The listing builds one solid part. Answer for the finished solid, in the listing's coordinates (mm). A direction names the side the tool comes from. Round coordinates to 2 decimals unless told otherwise and drop trailing zeros. Write each loop counter-clockwise with the first axis right and the second up, starting at its lowest first coordinate (ties: lowest second). Pieces come first, ordered by that corner, then holes. Notation, with made-up numbers: (89.5, -15) - (116.5, -15) arc R17 cw to (116.5, -3) - close; hole circle Ø10 at (24.25, -30). An arc over 180 degrees is marked (long way). Return JSON: item names as keys, results as strings. Group by question number.
(1) Which of the six approach directions +Z, -Z, +X, -X, +Y, -Y give full straight-line access (tool end or side, diameter ignored) to faces 1 (the cylindrical face through (17.161, 2.718, 4.213)), 2 (the cylindrical face through (-8.76, 1.535, -17.483)), 3 (the flat face through (-6, -1, 15))?
(2) Section A-A, the plane z = -22.5 is taken. Write down the section's boundary in (x, y).
(3) Determine the mould class of faces 4 (the flat face through (36, 0, 0)), 5 (the flat face through (-28, 0, 22)), 6 (the flat face through (-36, 0, 0)) for opening direction X: +X half, -X half, draft (parallel to the pull), parting line (faces both ways), or undercut.
(4) Section D-D, the plane z = 0 is taken. Write down the section's boundary in (x, y).
(5) Each of these flat-tipped pins is pushed along its axis until it touches: pin 1 (5.5 mm diameter, centred on x = 22.5, z = 15.5, fed in from -Y); pin 2 (2.5 mm diameter, centred on x = -32, z = -1, fed in from +Y); pin 3 (13 mm diameter, centred on x = -31, z = 22.5, fed in from +Y); pin 4 (6.5 mm diameter, centred on x = 3, z = -1.5, fed in from +Y). Where does it stop, or does it pass through?
(6) Find the intervals of material crossed by line 1 along Z through (x, y) = (-31, 2.85); line 2 along X through (y, z) = (2.1, -15.5); line 3 along Z through (x, y) = (-31, -1.3), in increasing order. Write a range as [from, to].
(7) Section C-C, the plane x = 7 is taken. Write down the section's boundary in (y, z), then the cut area to 3 significant figures.
(8) Section B-B, the plane y = -2 is taken. Give the number of separate pieces and of enclosed holes in the cut face, then the cut area to 3 significant figures.
```python
from build123d import *

# Parameters (mm, degrees)
SKETCH_1_W                = 72
SKETCH_1_H                = 65
EXTRUDE_1_DEPTH           = 4
HOLE_WIZARD_1_D           = 5.5
HOLE_WIZARD_1_DEPTH       = 100
HOLE_WIZARD_1_CBORE_D     = 22
HOLE_WIZARD_1_CBORE_DEPTH = 2.6
HOLE_WIZARD_2_D           = 4
HOLE_WIZARD_2_DEPTH       = 100
HOLE_WIZARD_2_CBORE_D     = 6
HOLE_WIZARD_2_CBORE_DEPTH = 3
HOLE_WIZARD_3_D           = 5
HOLE_WIZARD_3_DEPTH       = 100
HOLE_WIZARD_3_CBORE_D     = 8
HOLE_WIZARD_3_CBORE_DEPTH = 4
CHAMFER_1_SIZE            = 0.8


with BuildPart() as part:
    # 草图1 → 凸台-拉伸1 (new, symmetric)
    with BuildSketch(Plane(origin=(0, 0, 0), x_dir=(1, 0, 0), z_dir=(0, 1, 0))):
        Rectangle(SKETCH_1_W, SKETCH_1_H)
    extrude(amount=EXTRUDE_1_DEPTH, both=True)

    # 孔1
    with Locations(Plane(origin=(0, 4, 0), x_dir=(1, 0, 0), z_dir=(0, 1, 0))):
        with Locations((7, 0)):
            CounterBoreHole(HOLE_WIZARD_1_D / 2, HOLE_WIZARD_1_CBORE_D / 2, HOLE_WIZARD_1_CBORE_DEPTH, depth=HOLE_WIZARD_1_DEPTH)

    # 孔2
    with Locations(Plane(origin=(0, -4, 0), x_dir=(-1, 0, 0), z_dir=(0, -1, 0))):
        with Locations((-22.5, 15.5), (8.5, 15.5), (8.5, -15.5), (-22.5, -15.5)):
            CounterBoreHole(HOLE_WIZARD_2_D / 2, HOLE_WIZARD_2_CBORE_D / 2, HOLE_WIZARD_2_CBORE_DEPTH, depth=HOLE_WIZARD_2_DEPTH)

    # 孔3
    with Locations(Plane(origin=(0, 4, 0), x_dir=(1, 0, 0), z_dir=(0, 1, 0))):
        with Locations((-31, 22.5), (-31, 0), (-31, -22.5)):
            CounterBoreHole(HOLE_WIZARD_3_D / 2, HOLE_WIZARD_3_CBORE_D / 2, HOLE_WIZARD_3_CBORE_DEPTH, depth=HOLE_WIZARD_3_DEPTH)

    # 倒角1
    chamfer_1_edges = [part.edges().sort_by_distance(p)[0] for p in [
        (-36, 4, 0),
        (0, 4, 32.5),
        (36, 4, 0),
        (36, 0, 32.5),
        (-36, 0, 32.5),
        (-36, 0, -32.5),
        (36, 0, -32.5),
        (0, 4, -32.5),
    ]]
    chamfer(chamfer_1_edges, length=CHAMFER_1_SIZE)


solid = part.part
```
Working result:
{
 "1": {"face 1": "+Y", "face 2": "+Y, -Y", "face 3": "-Y"},
 "2": {"outline": "(-36, -4) - (-33.5, -4) - (-33.5, 0) - (-35, 0) - (-35, 4) - (-35.2, 4) - (-36, 3.2) - close; (-28.5, -4) - (36, -4) - (36, 3.2) - (35.2, 4) - (-27, 4) - (-27, 0) - (-28.5, 0) - close"},
 "3": {"face 4": "+X half", "face 5": "undercut", "face 6": "-X half"},
 "4": {"outline": "(-36, -4) - (-33.5, -4) - (-33.5, 0) - (-35, 0) - (-35, 4) - (-35.2, 4) - (-36, 3.2) - close; (-28.5, -4) - (4.25, -4) - (4.25, 1.4) - (-4, 1.4) - (-4, 4) - (-27, 4) - (-27, 0) - (-28.5, 0) - close; (9.75, -4) - (36, -4) - (36, 3.2) - (35.2, 4) - (18, 4) - (18, 1.4) - (9.75, 1.4) - close"},
 "5": {"pin 1": "stops at y = -1", "pin 2": "stops at y = 0", "pin 3": "stops at y = 4", "pin 4": "stops at y = 1.4"},
 "6": {"line 1": "z = [-32.5, -26.5], [-18.5, -4], [4, 18.5], [26.5, 32.5]", "line 2": "x = [-36, -10.5], [-6.5, 20.5], [24.5, 36]", "line 3": "z = [-32.5, -25], [-20, -2.5], [2.5, 20], [25, 32.5]"},
 "7": {"outline": "(-4, -32.5) - (3.2, -32.5) - (4, -31.7) - (4, -11) - (1.4, -11) - (1.4, -2.75) - (-4, -2.75) - close; (-4, 2.75) - (1.4, 2.75) - (1.4, 11) - (4, 11) - (4, 31.7) - (3.2, 32.5) - (-4, 32.5) - close", "area": "432 mm^2"},
 "8": {"separate pieces": "1", "enclosed holes": "8", "area": "4,480 mm^2"}
}
